The listing builds one solid part. Answer for the finished solid, in the listing's coordinates (mm). A direction names the side the tool comes from. Coordinates: 2 decimals unless noted, no trailing zeros. Order: outer loops, then holes, each group sorted by start corner. A loop starts at its lowest first (then second) coordinate and runs counter-clockwise, first axis right, second up.
from build123d import *

# Parameters (mm, degrees)
SKETCH1_W           = 56.4
SKETCH1_H           = 56.4
BOSS_EXTRUDE1_DEPTH = 78
FILLET1_R           = 3.5
SKETCH2_R           = 19.05
BOSS_EXTRUDE2_DEPTH = 1.6
SKETCH4_R           = 3.175
BOSS_EXTRUDE3_DEPTH = 20.6
SKETCH5_R           = 2.5
CUT_EXTRUDE1_DEPTH  = 112.561283607
CUT_EXTRUDE2_START  = -73.2
SKETCH8_R           = 5.5
CUT_EXTRUDE2_DEPTH  = 73.2
FILLET2_R           = 2


with BuildPart() as part:
    # Sketch1 → Boss-Extrude1 (new body)
    with BuildSketch(Plane.XY):
        with Locations((28.2, 28.2)):
            Rectangle(SKETCH1_W, SKETCH1_H)
    extrude(amount=BOSS_EXTRUDE1_DEPTH)

    # Fillet1
    fillet1_edges = [part.edges().sort_by_distance(p)[0] for p in [
        (0, 56.4, 39),
        (56.4, 56.4, 39),
        (56.4, 0, 39),
        (0, 0, 39),
    ]]
    fillet(fillet1_edges, radius=FILLET1_R)

    # Sketch2 → Boss-Extrude2 (add)
    with BuildSketch(Plane(origin=(0, 0, 0), x_dir=(-1, 0, 0), z_dir=(0, 0, -1))):
        with Locations(Location((-28.2, 28.2, 0), (0, 0, 180))):
            Circle(SKETCH2_R)
    extrude(amount=BOSS_EXTRUDE2_DEPTH)

    # Sketch4 → Boss-Extrude3 (add)
    with BuildSketch(Plane(origin=(0, 0, 0), x_dir=(-1, 0, 0), z_dir=(0, 0, -1))):
        with Locations(Location((-28.2, 28.2, 0), (0, 0, 180))):
            Circle(SKETCH4_R)
    extrude(amount=BOSS_EXTRUDE3_DEPTH)

    # Sketch5 → Cut-Extrude1 (cut, through all)
    with BuildSketch(Plane(origin=(0, 0, 0), x_dir=(-1, 0, 0), z_dir=(0, 0, -1))):
        with Locations((-51.77, 51.77)):
            Circle(SKETCH5_R)
        with Locations((-4.63, 51.77)):
            Circle(SKETCH5_R)
        with Locations((-4.63, 4.63)):
            Circle(SKETCH5_R)
        with Locations((-51.77, 4.63)):
            Circle(SKETCH5_R)
    extrude(amount=-CUT_EXTRUDE1_DEPTH, mode=Mode.SUBTRACT)

    # Sketch8 → Cut-Extrude2 (cut)
    with BuildSketch(Plane.XY.offset(78).offset(CUT_EXTRUDE2_START)):
        with Locations((4.63, 51.77)):
            Circle(SKETCH8_R)
        with Locations((51.77, 51.77)):
            Circle(SKETCH8_R)
        with Locations((51.77, 4.63)):
            Circle(SKETCH8_R)
        with Locations((4.63, 4.63)):
            Circle(SKETCH8_R)
    extrude(amount=CUT_EXTRUDE2_DEPTH, mode=Mode.SUBTRACT)

    # Fillet2
    fillet2_edges = [part.edges().sort_by_distance(p)[0] for p in [
        (0, 7.598686578, 41.4),
        (7.598686578, 0, 41.4),
        (0, 48.801313422, 41.4),
        (7.598686578, 56.4, 41.4),
        (56.4, 48.801313422, 41.4),
        (48.801313422, 56.4, 41.4),
        (48.801313422, 0, 41.4),
        (56.4, 7.598686578, 41.4),
    ]]
    fillet(fillet2_edges, radius=FILLET2_R)


solid = part.part
(1) Given pin 1 Ø6.5 at (x, y) = (51.77, 51.77) entering from +Z; pin 2 Ø6 at (x, y) = (4.63, 4.63) entering from -Z; pin 3 Ø12 at (x, y) = (22.5, 48.5) entering from -Z, each flat-ended and moving along its own axis, determine where each tip first touches the part or whether it passes through.
(2) Find section C-C on z = 2. Determine the outline of the cut face in (x, y).
(3) Find the intervals of material crossed by probe 1 along Y at (x, z) = (4.63, 3.45); probe 2 along X at (y, z) = (4, 2); probe 3 along X at (y, z) = (51, 3), in increasing order.
(4) Find section A-A on y = 4.63. Determine the outline of the cut face in (x, z).
(5) A tool of negligible diameter and unlimited length cuts with its end or side. For faces 1 (the cylindrical face through (8.58, 8.46, 40.89)), 2 (the cylindrical face through (0.883, 9.995, 40.888)), 3 (the cylindrical face through (25.72, 9.312, -0.789)), from which of +Z, -Z, +X, -X, +Y, -Y can it reach the whole face along a straight path? Write none if from no direction.
(6) Find section D-D on x = 28.2. Determine the outline of the cut face in (y, z) (3 decimals), then the cut area to 3 significant figures.
(7) The mould has two halves that part along X. Classify faces 4 (the cylindrical face through (46.405, 0.883, 40.888)), 5 (the cylindrical face through (8.46, 47.82, 40.89)), 6 (the cylindrical face through (25.68, 30.13, -10.97)): pulls with the +X half, pulls with the -X half, needs draft (parallel to the pull), parting line crosses it, or undercut.
Resolved:
1. pin 1: stops at z = 4.8
1. pin 2: stops at z = 0
1. pin 3: stops at z = -1.6
2. outline: (0, 3.5) arc R3.5 ccw to (3.5, 0) - (52.9, 0) arc R3.5 ccw to (56.4, 3.5) - (56.4, 52.9) arc R3.5 ccw to (52.9, 56.4) - (3.5, 56.4) arc R3.5 ccw to (0, 52.9) - close; hole circle Ø5 at (4.63, 4.63); hole circle Ø5 at (4.63, 51.77); hole circle Ø5 at (51.77, 4.63); hole circle Ø5 at (51.77, 51.77)
3. probe 1: y = 0 to 2.13, 7.13 to 49.27, 54.27 to 56.4
3. probe 2: x = 0 to 2.21, 7.05 to 49.35, 54.19 to 56.4
3. probe 3: x = 0 to 2.25, 7.01 to 49.39, 54.15 to 56.4
4. outline: (0, 0) - (2.13, 0) - (2.13, 4.8) - (0, 4.8) - close; (7.13, 0) - (49.27, 0) - (49.27, 4.8) - (46.27, 4.8) - (46.27, 78) - (10.13, 78) - (10.13, 4.8) - (7.13, 4.8) - close; (54.27, 0) - (56.4, 0) - (56.4, 4.8) - (54.27, 4.8) - close
5. face 1: +Z
5. face 2: +Z, -Y
5. face 3: -Z
6. outline: (0, 0) - (9.15, 0) - (9.15, -1.6) - (25.025, -1.6) - (25.025, -20.6) - (31.375, -20.6) - (31.375, -1.6) - (47.25, -1.6) - (47.25, 0) - (56.4, 0) - (56.4, 78) - (0, 78) - close
6. area: 4,580 mm2
7. face 4: pulls with the +X half
7. face 5: undercut
7. face 6: parting line crosses it
